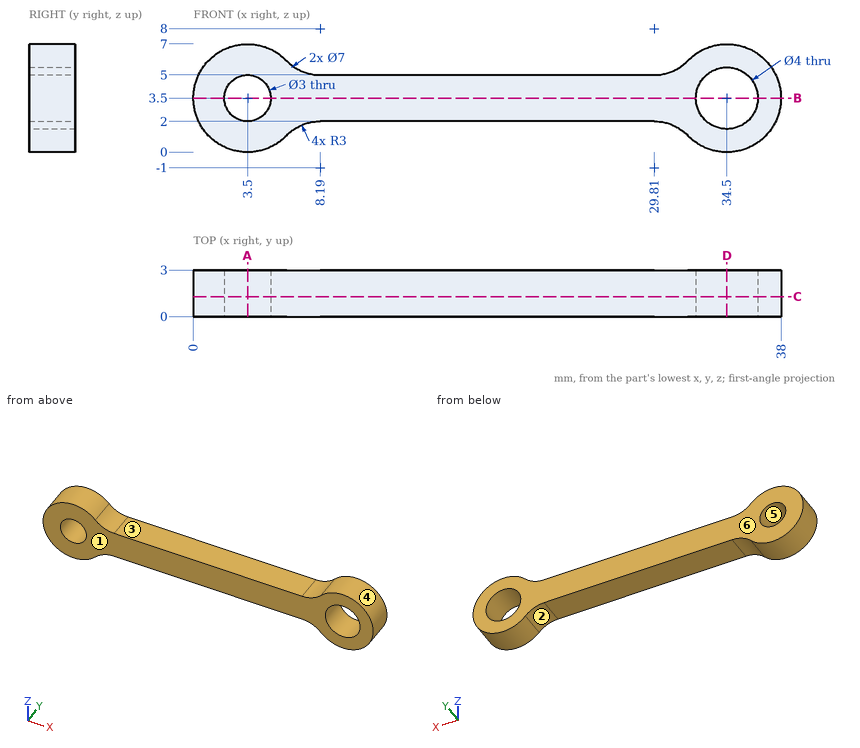
Here's the drawing with two shaded views (mm, measured from the low corner). I have some questions. A direction names the side the tool comes from. Give positions to 0.01 mm unless a question says otherwise; leave off trailing zeros. Order: outer loops, then holes, each group sorted by start corner. A loop starts at its lowest first (then second) coordinate and runs counter-clockwise, first axis right, second up. Notation, with made-up numbers: M -31.5,-38.75 L 19.5,-38.75 A12 ccw 19.5,-19.75 Z; hole C 30,89 d11. An arc over 180 degrees is marked long. One line per item, written item: value.
1) Please list where these lines run through material, in increasing order: line 1 along X through (y, z) = (2.05, 3.5); line 2 along Z through (x, y) = (30, 2.5); line 3 along X through (y, z) = (2.75, 3) (1 decimal).
Answer sheet:
line 1: x = 0 to 2, 5 to 32.5, 36.5 to 38
line 2: z = 1.99 to 5.01
line 3: x = 0 to 2.1, 4.9 to 32.6, 36.4 to 38
2) On a 3-axis mill with a long thin cutter (end or side, diameter ignored), from which of +Z, -Z, +X, -X, +Y, -Y can I reach the whole of each face in a straight line? I mean the marked faces 1, 2 and 3. Say none if no direction works.
Answer sheet:
face 1: +Z, -Z, +X, -X, -Y
face 2: -Z, +Y, -Y
face 3: +Z, +Y, -Y
3) For P1, Ø1.8, axis at x = 3.5, z = 3.5, coming from the +Y side; P2, Ø1.5, axis at x = 14, y = 1.5, coming from the -Z side; P3, Ø0.9, axis at x = 23.5, y = 2, coming from the +Z side, each with a flat end and sliding along its axis, tell me the tip position at first contact or that it passes through.
Answer sheet:
P1: passes through
P2: stops at z = 2
P3: stops at z = 5
4) I want a section at B-B, the plane z = 3.5. List the corners of the cut face in (x, y) for me.
Answer sheet:
outline: M 0,0 L 2,0 L 2,3 L 0,3 Z; M 5,0 L 32.5,0 L 32.5,3 L 5,3 Z; M 36.5,0 L 38,0 L 38,3 L 36.5,3 Z
5) I want a section at D-D, the plane x = 34.5. List the corners of the cut face in (y, z) for me.
Answer sheet:
outline: M 0,0 L 3,0 L 3,1.5 L 0,1.5 Z; M 0,5.5 L 3,5.5 L 3,7 L 0,7 Z
6) I want a section at C-C, the plane y = 1.3. List the corners of the cut face in (x, z) for me (1 decimal), plus the area to 3 significant figures.
Answer sheet:
outline: M 6,1.1 A3 cw 8.2,2 L 29.8,2 A3 cw 32,1.1 A3.5 ccw long 32,5.9 A3 cw 29.8,5 L 8.2,5 A3 cw 6,5.9 A3.5 ccw long Z; hole C 3.5,3.5 d3; hole C 34.5,3.5 d4
area: 131 mm^2
7) I want a section at A-A, the plane x = 3.5. List the corners of the cut face in (y, z) for me.
Answer sheet:
outline: M 0,0 L 3,0 L 3,2 L 0,2 Z; M 0,5 L 3,5 L 3,7 L 0,7 Z
8) We'd pull the mould along Z, two halves only. Please class the marked faces 4, 5 and 6: released by +Z, released by -Z, zero draft, split by the parting line, or undercut.
Answer sheet:
face 4: split by the parting line
face 5: undercut
face 6: zero draft
